Model file for the job. Use its own axes, mm. A direction names the side the tool comes from. Give positions to 0.01 mm unless a question says otherwise; leave off trailing zeros. Loops run counter-clockwise (first coordinate to the right, second up) from the corner with the lowest first, then second, coordinate; pieces in that order, holes last. Notation, with made-up numbers: M 57.25,12.5 L 107.25,12.5 A13 cw 107.25,19.5 Z; hole C -9.5,25.5 d9. An arc over 180 degrees is marked long. Answer in a Markdown table with one row per item.
```python
from build123d import *

# Parameters (mm, degrees)
BOSS_EXTRUDE2_DEPTH      = 50
BOSS_EXTRUDE2_DEPTH_BACK = 50
SKETCH4_W                = 330
SKETCH4_H                = 25
SKETCH5_R                = 32.5
CUT_EXTRUDE1_DEPTH       = 215.413152582


with BuildPart() as part:
    # Sketch1 → Boss-Extrude2 (new, two sides: drawn at the far end of the back side and taken through both)
    with BuildSketch(Plane.XY.offset(-BOSS_EXTRUDE2_DEPTH_BACK)):
        Polygon((0, -93.530743609), (81, -46.765371804), (81, 46.765371804), (0, 93.530743609), (-81, 46.765371804), (-81, -46.765371804), align=None)
    extrude(amount=BOSS_EXTRUDE2_DEPTH + BOSS_EXTRUDE2_DEPTH_BACK)

    # Sketch4 → Revolve2 (revolve)
    with BuildSketch(Plane.XY):
        with Locations((0, 12.5)):
            Rectangle(SKETCH4_W, SKETCH4_H)
    revolve(axis=Axis((165, 0, 0), (-1, 0, 0)))

    # Sketch5 → Cut-Extrude1 (cut, through all)
    with BuildSketch(Plane.XY.offset(50)):
        Circle(SKETCH5_R)
    extrude(amount=-CUT_EXTRUDE1_DEPTH, mode=Mode.SUBTRACT)


solid = part.part
```
Q1. Drop flat-ended pins along their axis: pin 1 (2 mm diameter, centred on x = -86.5, z = 16, fed in from -Y); pin 2 (5 mm diameter, centred on x = -104.5, z = -5.5, fed in from -Y); pin 3 (2 mm diameter, centred on x = 59, z = -39.5, fed in from -Y). Give the stop position or say it passes through.
Reported:
| item | result |
|---|---|
| pin 1 | y = -20 |
| pin 2 | y = -24.82 |
| pin 3 | y = -60.04 |
Q2. Saw through at D-D (x = 37). Give the cut face in (y, z), and give its area (3 significant figures).
Reported:
| item | result |
|---|---|
| outline | M -72.17,-50 L 72.17,-50 L 72.17,50 L -72.17,50 Z |
| area | 14,400 mm² |
Q3. Saw through at C-C (z = 0). Give the cut face in (x, y).
Reported:
| item | result |
|---|---|
| outline | M -165,-25 L -81,-25 L -81,-46.77 L 0,-93.53 L 81,-46.77 L 81,-25 L 165,-25 L 165,25 L 81,25 L 81,46.77 L 0,93.53 L -81,46.77 L -81,25 L -165,25 Z; hole C 0,0 d65 |
Q4. Saw through at B-B (z = 43). Give the cut face in (x, y), and give its area (3 significant figures).
Reported:
| item | result |
|---|---|
| outline | M -81,-46.77 L 0,-93.53 L 81,-46.77 L 81,46.77 L 0,93.53 L -81,46.77 Z; hole C 0,0 d65 |
| area | 19,400 mm² |
Q5. Mould opens along X. For faces 1 (the face through (-81, 11, -23)), 2 (the face through (-1, -40, 50)), 3 (the face through (31, 9.76, 0.7)) say: released by +X, released by -X, zero draft, split by the parting line, or undercut.
Reported:
| item | result |
|---|---|
| face 1 | released by -X |
| face 2 | zero draft |
| face 3 | undercut |
Q6. 3-axis set-ups, long thin cutter, end or side, ignore diameter. For faces 4 (the face through (-41.1, -69.8, -0.7)), 5 (the face through (-122.412, 23.846, -7.509)), 6 (the face through (81, -11, -23)): which of +Z, -Z, +X, -X, +Y, -Y reach the whole face in a straight line?
Reported:
| item | result |
|---|---|
| face 4 | +Z, -Z, -X, -Y |
| face 5 | -X |
| face 6 | +X |
Q7. Probe probe 1 along X at (y, z) = (1.5, -7.5); probe 2 along Y at (x, z) = (0, 1.5); probe 3 along X at (y, z) = (-18.5, 13). List the from-to ranges inside material, lowest first.
Reported:
| item | result |
|---|---|
| probe 1 | -165 to -32.47, 32.47 to 165 |
| probe 2 | -93.53 to -32.5, 32.5 to 93.53 |
| probe 3 | -165 to -26.72, 26.72 to 165 |
Q8. Saw through at A-A (y = 0). Give the cut face in (x, z), and give its area (3 significant figures).
Reported:
| item | result |
|---|---|
| outline | M -165,-25 L -81,-25 L -81,-50 L -32.5,-50 L -32.5,50 L -81,50 L -81,25 L -165,25 Z; M 32.5,-50 L 81,-50 L 81,-25 L 165,-25 L 165,25 L 81,25 L 81,50 L 32.5,50 Z |
| area | 18,100 mm² |
